from build123d import *

# Parameters (mm, degrees)
RESSALTO_EXTRUS_O1_DEPTH   = 3
ESBO_O2_W                  = 12
ESBO_O2_H                  = 3
CORTE_EXTRUS_O1_DEPTH      = 59.67394737
FURO_DE_DI_METRO_3_0_3_1_D = 3
ESBO_O5_W                  = 3
ESBO_O5_H                  = 6
ESBO_O5_H_2                = 3
ESBO_O5_W_2                = 6
ESBO_O5_H_3                = 9
ESBO_O5_W_3                = 10
RESSALTO_EXTRUS_O2_DEPTH   = 3


with BuildPart() as part:
    # Esboço1 → Ressalto-extrusão1 (new body)
    with BuildSketch(Plane.XY):
        with BuildLine():
            Line((0, 0), (48, 0))
            Line((48, 0), (48, 24.75))
            ThreePointArc((48, 24.75), (40.90916402, 33.431570058), (30.986533031, 28.217070289))
            ThreePointArc((30.986533031, 28.217070289), (21.771923029, 17.148462374), (7.980136393, 13))
            Line((7.980136393, 13), (0, 13))
            Line((0, 13), (0, 0))
        make_face()
    extrude(amount=-RESSALTO_EXTRUS_O1_DEPTH)

    # Esboço2 → Corte-extrusão1 (cut, through all)
    with BuildSketch(Plane.XY):
        with Locations((24, 1.5)):
            Rectangle(ESBO_O2_W, ESBO_O2_H)
    extrude(amount=-CORTE_EXTRUS_O1_DEPTH, mode=Mode.SUBTRACT)

    # Furo de diâmetro Ø3.0 (3)1 (through all)
    with Locations(Plane.XY):
        with Locations((39.14, 24.75)):
            Hole(FURO_DE_DI_METRO_3_0_3_1_D / 2)

    # Esboço5 → Ressalto-extrusão2 (add, through all)
    with BuildSketch(Plane.XY):
        with Locations((-1.5, 3)):
            Rectangle(ESBO_O5_W, ESBO_O5_H)
        with Locations((1.5, -1.5)):
            Rectangle(ESBO_O5_W, ESBO_O5_H_2)
        with Locations((7.5, -1.5)):
            Rectangle(ESBO_O5_W_2, ESBO_O5_H_2)
        with Locations((49.5, 4.5)):
            Rectangle(ESBO_O5_W, ESBO_O5_H_3)
        with Locations((43, -1.5)):
            Rectangle(ESBO_O5_W_3, ESBO_O5_H_2)
    extrude(amount=-RESSALTO_EXTRUS_O2_DEPTH)


solid = part.part
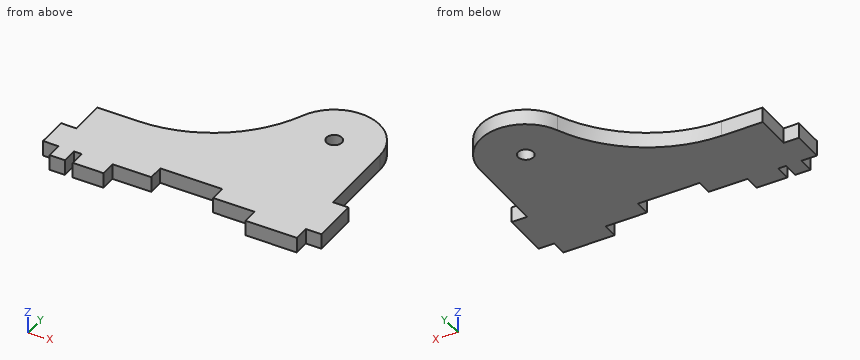
Input: part model. Units: mm. Frame: model coordinates. Give positions to 0.01 mm unless a question says otherwise; leave off trailing zeros. Write each loop counter-clockwise with the first axis right and the second up, starting at its lowest first coordinate (ties: lowest second). Pieces come first, ordered by that corner, then holes.
Q1. First-contact query: P1, Ø4, axis at x = 13.5, y = 7.5, coming from the +Z side; P2, Ø0.9, axis at y = -2, z = -1.5, coming from the +X side. Flat tips, straight axial feed; report the tip coordinate or a pass-through.
Q2. Section B-B, the plane x = 39.14. Output: boundary loops of the cut face in (y, z), plus the area to 3 significant figures.
Q3. Section C-C, the plane y = 12. Output: boundary loops of the cut face in (x, z), plus the area to 3 significant figures.
Q4. Material intervals for probe 1 along X at (y, z) = (-1, -0.4); probe 2 along Y at (x, z) = (39.14, -2.25); probe 3 along X at (y, z) = (0.5, -0.95), sorted ascending.
Q5. Section A-A, the plane z = -1.3. Output: boundary loops of the cut face in (x, y), plus the area to 3 significant figures.
Q6. Section D-D, the plane x = 2. Output: boundary loops of the cut face in (y, z), plus the area to 3 significant figures.
Filled in:
1. P1: stops at z = 0
1. P2: stops at x = 48
2. outline: (-3, -3) - (23.25, -3) - (23.25, 0) - (-3, 0) - close; (26.25, -3) - (33.61, -3) - (33.61, 0) - (26.25, 0) - close
2. area: 101 mm2
3. outline: (0, -3) - (48, -3) - (48, 0) - (0, 0) - close
3. area: 144 mm2
4. probe 1: x = 0 to 3, 4.5 to 10.5, 38 to 48
4. probe 2: y = -3 to 23.25, 26.25 to 33.61
4. probe 3: x = -3 to 18, 30 to 51
5. outline: (-3, 0) - (0, 0) - (0, -3) - (3, -3) - (3, 0) - (4.5, 0) - (4.5, -3) - (10.5, -3) - (10.5, 0) - (18, 0) - (18, 3) - (30, 3) - (30, 0) - (38, 0) - (38, -3) - (48, -3) - (48, 0) - (51, 0) - (51, 9) - (48, 9) - (48, 24.75) arc R8.86 ccw to (30.99, 28.22) arc R25 cw to (7.98, 13) - (0, 13) - (0, 6) - (-3, 6) - close; hole circle Ø3 at (39.14, 24.75)
5. area: 1,100 mm2
6. outline: (-3, -3) - (13, -3) - (13, 0) - (-3, 0) - close
6. area: 48.0 mm2
